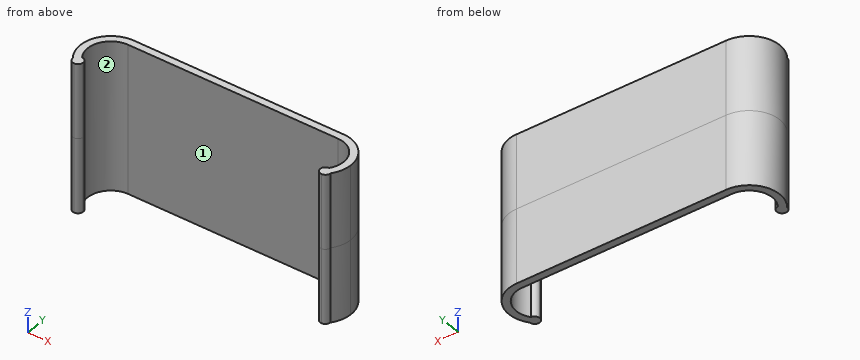
from build123d import *

# Parameters (mm, degrees)
F1_DEPTH = 20


with BuildPart() as f1:
    # F0 (on Top) → F1 (new body, symmetric)
    with BuildSketch(Plane.XY):
        with BuildLine():
            Line((-28.75, 8.25), (-28.75, 6.25))
            Line((-28.75, 6.25), (-23.3648351929, 6.25))
            ThreePointArc((-23.3648351929, 6.25), (-25.8777186767, 7.7338541491), (-28.75, 8.25))
        make_face()
        with BuildLine():
            ThreePointArc((-33.8628873162, -3.5945630182), (-34.2965538339, 2.8806666881), (-28.75, 6.25))
            Line((-28.75, 6.25), (-28.75, 8.25))
            ThreePointArc((-28.75, 8.25), (-36.1429865413, 3.661454629), (-35.3122023742, -5))
            ThreePointArc((-35.3122023742, -5), (-34.8849672334, -3.9905735233), (-33.8628873162, -3.5945630182))
        make_face()
        with BuildLine():
            ThreePointArc((-28.75, 8.25), (-25.8777186767, 7.7338541491), (-23.3648351929, 6.25))
            Line((-23.3648351929, 6.25), (23.3648351929, 6.25))
            ThreePointArc((23.3648351929, 6.25), (25.8777186767, 7.7338541491), (28.75, 8.25))
            Line((28.75, 8.25), (-28.75, 8.25))
        make_face()
        with BuildLine():
            ThreePointArc((-32.5, -5), (-32.8966747104, -4.0211339537), (-33.8628873162, -3.5945630182))
            ThreePointArc((-33.8628873162, -3.5945630182), (-33.2368147022, -4.3509761925), (-32.5, -5))
        make_face()
        with BuildLine():
            ThreePointArc((-32.5, -5), (-33.2368147022, -4.3509761925), (-33.8628873162, -3.5945630182))
            ThreePointArc((-33.8628873162, -3.5945630182), (-34.8849672334, -3.9905735233), (-35.3122023742, -5))
            Line((-35.3122023742, -5), (-32.5, -5))
        make_face()
        with BuildLine():
            ThreePointArc((28.75, 8.25), (25.8777186767, 7.7338541491), (23.3648351929, 6.25))
            Line((23.3648351929, 6.25), (28.75, 6.25))
            Line((28.75, 6.25), (28.75, 8.25))
        make_face()
        with BuildLine():
            ThreePointArc((-33.949315058, -6.4054369818), (-32.9272351408, -6.0094264767), (-32.5, -5))
            Line((-32.5, -5), (-35.3122023742, -5))
            ThreePointArc((-35.3122023742, -5), (-34.672595407, -5.7432885741), (-33.949315058, -6.4054369818))
        make_face()
        with BuildLine():
            ThreePointArc((37, 0), (34.5836309448, 5.8336309448), (28.75, 8.25))
            Line((28.75, 8.25), (28.75, 6.25))
            ThreePointArc((28.75, 6.25), (33.1694173824, 4.4194173824), (35, 0))
            ThreePointArc((35, 0), (34.7089447776, -1.8850668786), (33.8628873162, -3.5945630182))
            ThreePointArc((33.8628873162, -3.5945630182), (34.8849672334, -3.9905735233), (35.3122023742, -5))
            ThreePointArc((35.3122023742, -5), (36.5666703137, -2.6385915194), (37, 0))
        make_face()
        with BuildLine():
            ThreePointArc((-33.949315058, -6.4054369818), (-34.672595407, -5.7432885741), (-35.3122023742, -5))
            ThreePointArc((-35.3122023742, -5), (-34.9155276638, -5.9788660463), (-33.949315058, -6.4054369818))
        make_face()
        with BuildLine():
            ThreePointArc((33.949315058, -6.4054369818), (34.9155276638, -5.9788660463), (35.3122023742, -5))
            ThreePointArc((35.3122023742, -5), (34.672595407, -5.7432885741), (33.949315058, -6.4054369818))
        make_face()
        with BuildLine():
            ThreePointArc((33.949315058, -6.4054369818), (34.672595407, -5.7432885741), (35.3122023742, -5))
            Line((35.3122023742, -5), (32.5, -5))
            ThreePointArc((32.5, -5), (32.9272351408, -6.0094264767), (33.949315058, -6.4054369818))
        make_face()
        with BuildLine():
            Line((32.5, -5), (35.3122023742, -5))
            ThreePointArc((35.3122023742, -5), (34.8849672334, -3.9905735233), (33.8628873162, -3.5945630182))
            ThreePointArc((33.8628873162, -3.5945630182), (33.2368147022, -4.3509761925), (32.5, -5))
        make_face()
        with BuildLine():
            ThreePointArc((33.8628873162, -3.5945630182), (32.8966747104, -4.0211339537), (32.5, -5))
            ThreePointArc((32.5, -5), (33.2368147022, -4.3509761925), (33.8628873162, -3.5945630182))
        make_face()
    extrude(amount=F1_DEPTH, both=True)


solid = f1.part
Geometry check sheet. Reference: the model listing, model coordinates, mm. Face numbers are marked on the shaded views. Coordinates: 2 decimals unless noted, no trailing zeros. Order: outer loops, then holes, each group sorted by start corner. A loop starts at its lowest first (then second) coordinate and runs counter-clockwise, first axis right, second up. Notation, with made-up numbers: (6, -6.5) - (52, -6.5) arc R20 ccw to (52, 19.5) - close; hole circle Ø1 at (-6.5, 74.5). An arc over 180 degrees is marked (long way). One line per item, written item: value.
(1) Sectioned sample at D-D (y = 3.5). Enter the section's corners in (x, z), and give its area (3 significant figures).
Data:
outline: (-36.22, -20) - (-33.93, -20) - (-33.93, 20) - (-36.22, 20) - close; (33.93, -20) - (36.22, -20) - (36.22, 20) - (33.93, 20) - close
area: 183 mm^2
(2) Sectioned sample at C-C (x = 4.5). Enter the section's corners in (y, z), and give its area (3 significant figures).
Data:
outline: (6.25, -20) - (8.25, -20) - (8.25, 20) - (6.25, 20) - close
area: 80.0 mm^2
(3) Thickness scan on probe 1 along Y at (x, z) = (6.5, -15); probe 2 along X at (y, z) = (3, -15); probe 3 along X at (y, z) = (5.75, -8). Record the ranges inside material, lowest first. Write a range as from..to.
Data:
probe 1: y = 6.25..8.25
probe 2: x = -36.44..-34.23, 34.23..36.44
probe 3: x = -34.67..-31.2, 31.2..34.67
(4) Sectioned sample at A-A (y = -0.75). Enter the section's corners in (x, z).
Data:
outline: (-36.97, -20) - (-34.95, -20) - (-34.95, 20) - (-36.97, 20) - close; (34.95, -20) - (36.97, -20) - (36.97, 20) - (34.95, 20) - close
(5) Depth check by flat-ended pin: pin 1 Ø4 at (y, z) = (1, 10.5) entering from -X; pin 2 Ø1 at (x, z) = (-0.5, -2.5) entering from -Y; pin 3 Ø1.5 at (y, z) = (-1.5, 9.5) entering from +X; pin 4 Ø8 at (x, y) = (-7, 1) entering from +Z. Enter the tip coordinate at first touch or a pass-through.
Data:
pin 1: stops at x = -37
pin 2: stops at y = 6.25
pin 3: stops at x = 36.97
pin 4: passes through
(6) Sectioned sample at B-B (z = -15.5). Enter the section's corners in (x, y).
Data:
outline: (-35.31, -5) arc R1.41 ccw (long way) to (-33.86, -3.59) arc R6.25 cw to (-28.75, 6.25) - (28.75, 6.25) arc R6.25 cw to (33.86, -3.59) arc R1.41 ccw (long way) to (35.31, -5) arc R8.25 ccw to (28.75, 8.25) - (-28.75, 8.25) arc R8.25 ccw to start
(7) Release check for a two-part mould opening along Y. For the marked faces 1 and 2 record: +Y half, -Y half, draft (parallel to the pull), parting line (faces both ways), or undercut.
Data:
face 1: -Y half
face 2: undercut
